```python
from build123d import *

# Parameters (mm, degrees)
CROQUIS1_R              = 9.5
CROQUIS1_R_2            = 4
SALIENTE_EXTRUIR1_DEPTH = 6
CROQUIS2_R              = 8.3
CROQUIS2_R_2            = 5.2
CORTAR_EXTRUIR1_DEPTH   = 0.1
REDONDEO1_R             = 0.3


with BuildPart() as part:
    # Croquis1 → Saliente-Extruir1 (new body)
    with BuildSketch(Plane(origin=(0, 0, 0), x_dir=(1, 0, 0), z_dir=(0, 1, 0))):
        with Locations(Location((0, 0, 0), (0, 0, 270))):
            Circle(CROQUIS1_R)
        with Locations(Location((0, 0, 0), (0, 0, 270))):
            Circle(CROQUIS1_R_2, mode=Mode.SUBTRACT)
    extrude(amount=SALIENTE_EXTRUIR1_DEPTH)

    # Croquis2 → Cortar-Extruir1 (cut)
    with BuildSketch(Plane(origin=(0, 6, 0), x_dir=(1, 0, 0), z_dir=(0, 1, 0))):
        with Locations(Location((0, 0, 0), (0, 0, 270))):
            Circle(CROQUIS2_R)
        with Locations(Location((0, 0, 0), (0, 0, 270))):
            Circle(CROQUIS2_R_2, mode=Mode.SUBTRACT)
    cortar_extruir1 = extrude(amount=-CORTAR_EXTRUIR1_DEPTH, mode=Mode.SUBTRACT)

    # Simetría1: Cortar-Extruir1 across plane
    add(cortar_extruir1.mirror(Plane.ZX.offset(3)), mode=Mode.SUBTRACT)

    # Redondeo1
    redondeo1_edges = [part.edges().sort_by_distance(p)[0] for p in [
        (0, 0, -9.5),
        (0, 6, -9.5),
        (0, 0, -4),
        (0, 6, -4),
    ]]
    fillet(redondeo1_edges, radius=REDONDEO1_R)


solid = part.part
```
CAD build for the part. Positions are in the model's coordinates, mm. A direction names the side the tool comes from. Round coordinates to 2 decimals unless told otherwise and drop trailing zeros. Write each loop counter-clockwise with the first axis right and the second up, starting at its lowest first coordinate (ties: lowest second). Pieces come first, ordered by that corner, then holes. Notation, with made-up numbers: (-29, -18.75) - (8, -18.75) arc R21 ccw to (8, 16.25) - close; hole circle Ø8 at (-14, 15). An arc over 180 degrees is marked (long way). Return JSON: item names as keys, results as strings. Group by question number.
Item 1: 3-axis set-ups, long thin cutter, end or side, ignore diameter. For faces 1 (the face through (4, 0, -2)), 2 (the face through (-4, 5.9, -4)): which of +Z, -Z, +X, -X, +Y, -Y reach the whole face in a straight line?
Item 2: Probe probe 1 along X at (y, z) = (0.4, 0); probe 2 along Y at (x, z) = (-5.25, 0.5); probe 3 along X at (y, z) = (5, 3.25). List the from-to ranges inside material, lowest first.
Item 3: Band-saw the part on C-C on y = 1.75. List the corners of the cut face in (x, z).
Item 4: Mould opens along Z. For faces 3 (the face through (-5.78, 2.96, -7.54)), 4 (the face through (7, 0, -5)), 5 (the face through (-4, 0.1, -4)) say: +Z half, -Z half, draft (parallel to the pull), parting line (faces both ways), or undercut.
Item 5: Flat gauge pins, fed straight in: pin 1 Ø1 at (x, y) = (-5, 0.5) entering from +Z; pin 2 Ø1.5 at (y, z) = (4.5, 7.5) entering from +X; pin 3 Ø6.5 at (x, z) = (0, 0) entering from +Y; pin 4 Ø1 at (y, z) = (0.5, -2.5) entering from -X. Where does each tip first touch, or does it go through?
Resolved:
{
 "1": {"face 1": "+Z, -Z, +X, -X, -Y", "face 2": "+Y"},
 "2": {"probe 1": "x = -9.5 to -4, 4 to 9.5", "probe 2": "y = 0.1 to 5.9", "probe 3": "x = -8.93 to -2.33, 2.33 to 8.93"},
 "3": {"outline": "circle Ø19 at (0, 0); hole circle Ø8 at (0, 0)"},
 "4": {"face 3": "parting line", "face 4": "draft", "face 5": "undercut"},
 "5": {"pin 1": "stops at z = 8.37", "pin 2": "stops at x = 6.68", "pin 3": "passes through", "pin 4": "stops at x = -9.29"}
}
